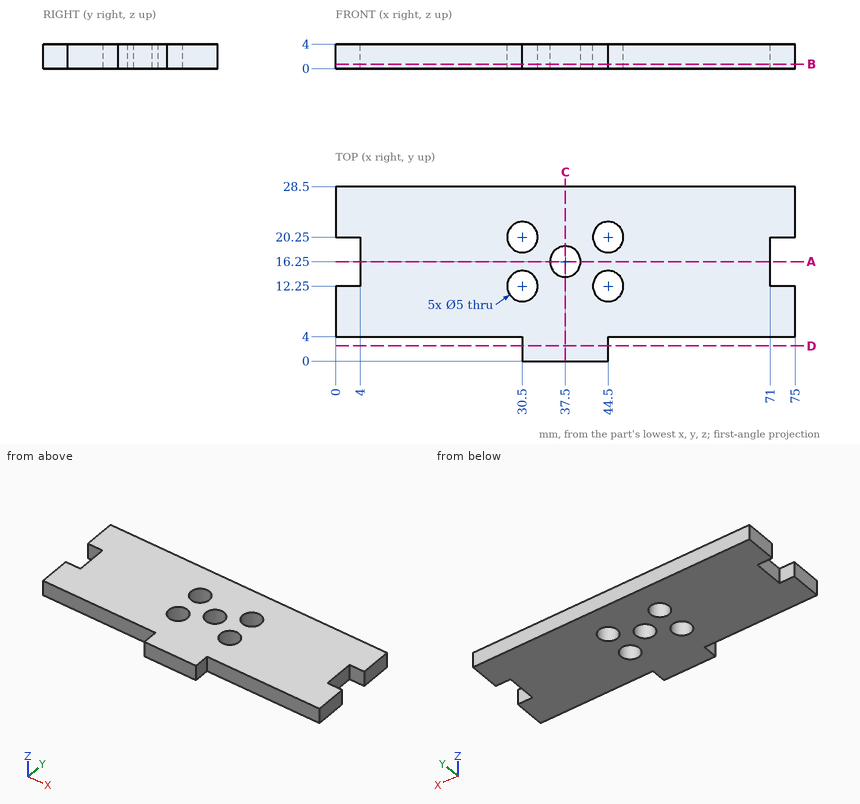
For this review, use the dimensioned drawing (mm, ordinates from the lowest corner) and the shaded views. Round coordinates to 2 decimals unless told otherwise and drop trailing zeros. Order: outer loops, then holes, each group sorted by start corner. A loop starts at its lowest first (then second) coordinate and runs counter-clockwise, first axis right, second up. Notation, with made-up numbers: M -22.5,-8.5 L 5.5,-8.5 A18 cw 5.5,3.5 Z; hole C 13,46.5 d1. An arc over 180 degrees is marked long. Use a Markdown table: item, result. Add a question column.
Item 1: Add section C-C, the plane x = 37.5. Give the boundary of the cut face in (y, z).
Item 2: Add section B-B, the plane z = 0.7. Give the boundary of the cut face in (x, y).
Item 3: Insertion check: pin 1 (2 mm diameter, centred on x = 12.5, z = 1, fed in from -Y); pin 2 (1.5 mm diameter, centred on x = 33, z = 1.5, fed in from -Y); pin 3 (1.2 mm diameter, centred on y = 1.5, z = 2, fed in from -X); pin 4 (1.2 mm diameter, centred on y = 16, z = 3, fed in from +X). Each pin has a flat end and moves straight along its axis. Give the tip position at first contact, or say it passes through.
Item 4: Add section A-A, the plane y = 16.25. Give the boundary of the cut face in (x, z), then the cut area to 3 significant figures.
Item 5: Add section D-D, the plane y = 2.5. Give the boundary of the cut face in (x, z).
Item 6: To check wall thickness, follow line 1 along X through (y, z) = (22, 1.4); line 2 along Y through (x, z) = (29.5, 1.15); line 3 along Y through (x, z) = (44, 1.75). State the ranges of each line that lie inside material, in increasing order.
Geometry results:
| question | item | result |
|---|---|---|
| 1 | outline | M 0,0 L 13.75,0 L 13.75,4 L 0,4 Z; M 18.75,0 L 28.5,0 L 28.5,4 L 18.75,4 Z |
| 2 | outline | M 0,4 L 30.5,4 L 30.5,0 L 44.5,0 L 44.5,4 L 75,4 L 75,12.25 L 71,12.25 L 71,20.25 L 75,20.25 L 75,28.5 L 0,28.5 L 0,20.25 L 4,20.25 L 4,12.25 L 0,12.25 Z; hole C 30.5,12.25 d5; hole C 30.5,20.25 d5; hole C 37.5,16.25 d5; hole C 44.5,12.25 d5; hole C 44.5,20.25 d5 |
| 3 | pin 1 | stops at y = 4 |
| 3 | pin 2 | stops at y = 0 |
| 3 | pin 3 | stops at x = 30.5 |
| 3 | pin 4 | stops at x = 71 |
| 4 | outline | M 4,0 L 35,0 L 35,4 L 4,4 Z; M 40,0 L 71,0 L 71,4 L 40,4 Z |
| 4 | area | 248 mm² |
| 5 | outline | M 30.5,0 L 44.5,0 L 44.5,4 L 30.5,4 Z |
| 6 | line 1 | x = 0 to 28.71, 32.29 to 42.71, 46.29 to 75 |
| 6 | line 2 | y = 4 to 9.96, 14.54 to 17.96, 22.54 to 28.5 |
| 6 | line 3 | y = 0 to 9.8, 14.7 to 17.8, 22.7 to 28.5 |
